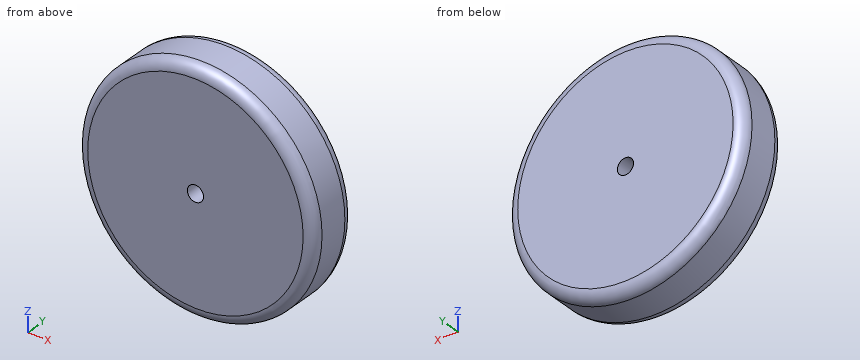
```python
from build123d import *

# Parameters (mm, degrees)
SKETCH1_R           = 69.85
BOSS_EXTRUDE1_DEPTH = 15.24
SKETCH2_R           = 4.7625
CUT_EXTRUDE1_DEPTH  = 30.48
FILLET1_R           = 6.35


with BuildPart() as part:
    # Sketch1 → Boss-Extrude1 (new body, symmetric)
    with BuildSketch(Plane(origin=(0, 0, 0), x_dir=(1, 0, 0), z_dir=(0, 1, 0))):
        Circle(SKETCH1_R)
    extrude(amount=BOSS_EXTRUDE1_DEPTH, both=True)

    # Sketch2 → Cut-Extrude1 (cut)
    with BuildSketch(Plane(origin=(0, 15.24, 0), x_dir=(1, 0, 0), z_dir=(0, 1, 0))):
        Circle(SKETCH2_R)
    extrude(amount=-CUT_EXTRUDE1_DEPTH, mode=Mode.SUBTRACT)

    # Fillet1
    fillet1_edges = [part.edges().sort_by_distance(p)[0] for p in [
        (-69.85, -15.24, 0),
        (-69.85, 15.24, 0),
    ]]
    fillet(fillet1_edges, radius=FILLET1_R)


solid = part.part
```
The listing builds one solid part. Answer for the finished solid, in the listing's coordinates (mm). Coordinates: 2 decimals unless noted, no trailing zeros. Write each loop counter-clockwise with the first axis right and the second up, starting at its lowest first coordinate (ties: lowest second). Pieces come first, ordered by that corner, then holes. Notation, with made-up numbers: (50, -12) - (78, -12) arc R12 cw to (78, 6) - close; hole circle Ø9 at (63.25, -23). An arc over 180 degrees is marked (long way). One line per item, written item: value.
1) Consider line 1 along X through (y, z) = (8, 0); line 2 along Y through (x, z) = (27.5, 57.5). Determine where each line is inside the solid, lowest interval first. Write a range as from..to.
Geometry check:
line 1: x = -69.85..-4.76, 4.76..69.85
line 2: y = -15.24..15.24
2) Find section A-A (x = 0). Give the vertices of the cut face in (y, z).
Geometry check:
outline: (-15.24, -63.5) arc R6.35 ccw to (-8.89, -69.85) - (8.89, -69.85) arc R6.35 ccw to (15.24, -63.5) - (15.24, -4.76) - (-15.24, -4.76) - close; (-15.24, 4.76) - (15.24, 4.76) - (15.24, 63.5) arc R6.35 ccw to (8.89, 69.85) - (-8.89, 69.85) arc R6.35 ccw to (-15.24, 63.5) - close
3) Find section B-B (z = 0). Give the vertices of the cut face in (x, y), and give its area (3 significant figures).
Geometry check:
outline: (-69.85, -8.89) arc R6.35 ccw to (-63.5, -15.24) - (-4.76, -15.24) - (-4.76, 15.24) - (-63.5, 15.24) arc R6.35 ccw to (-69.85, 8.89) - close; (4.76, -15.24) - (63.5, -15.24) arc R6.35 ccw to (69.85, -8.89) - (69.85, 8.89) arc R6.35 ccw to (63.5, 15.24) - (4.76, 15.24) - close
area: 3,930 mm2
4) Find section D-D (y = 11). Give the vertices of the cut face in (x, z) (1 decimal), and give its area (3 significant figures).
Geometry check:
outline: circle Ø139 at (0, 0); hole circle Ø9.5 at (0, 0)
area: 15,100 mm2
5) Each of these flat-tipped pins is pushed along its axis until it touches: pin 1 Ø8 at (x, y) = (-28, 7.5) entering from +Z; pin 2 Ø6 at (y, z) = (-11, 9.5) entering from +X; pin 3 Ø10 at (y, z) = (-12, -26.5) entering from -X. Where does it stop, or does it pass through?
Geometry check:
pin 1: stops at z = 65.6
pin 2: stops at x = 69.48
pin 3: stops at x = -66.22
